from build123d import *

# Parameters (mm, degrees)
BOSS_EXTRUDE1_DEPTH = 101.6
CUT_EXTRUDE1_START  = -25.4
SKETCH3_W           = 165.1
SKETCH3_H           = 76.2
CUT_EXTRUDE1_DEPTH  = 50.8
BOSS_EXTRUDE2_REACH = 306.27
SKETCH6_R           = 6.35


with BuildPart() as part:
    # Sketch1 → Boss-Extrude1 (new body)
    with BuildSketch(Plane.XY):
        with BuildLine():
            Line((0, 38.1), (254, 38.1))
            ThreePointArc((254, 38.1), (292.1, 0), (254, -38.1))
            Line((254, -38.1), (0, -38.1))
            ThreePointArc((0, -38.1), (-38.1, 0), (0, 38.1))
        make_face()
    extrude(amount=BOSS_EXTRUDE1_DEPTH)

    # Sketch3 → Cut-Extrude1 (cut)
    with BuildSketch(Plane.XY.offset(101.6).offset(CUT_EXTRUDE1_START)):
        Rectangle(SKETCH3_W, SKETCH3_H)
    cut_extrude1 = extrude(amount=-CUT_EXTRUDE1_DEPTH, mode=Mode.SUBTRACT)

    # Mirror1: Cut-Extrude1 across plane
    add(cut_extrude1.mirror(Plane(origin=(127, 0, 0), x_dir=(0, 0, 1), z_dir=(1, 0, 0))), mode=Mode.SUBTRACT)

    # Sketch6 → Boss-Extrude2 (add, up to next)
    with BuildSketch(Plane.XY.offset(25.4), mode=Mode.PRIVATE) as boss_extrude2_sk1:
        with Locations(Location((0, 0, 0), (0, 0, 180))):
            Circle(SKETCH6_R)
    boss_extrude2_tool1 = extrude(boss_extrude2_sk1.sketch, amount=BOSS_EXTRUDE2_REACH, mode=Mode.PRIVATE) - part.part
    boss_extrude2 = boss_extrude2_tool1.solids().sort_by_distance((0, 0, 25.4))[0]
    add(boss_extrude2)

    # Mirror2: Boss-Extrude2 across plane
    add(boss_extrude2.mirror(Plane(origin=(127, 0, 0), x_dir=(0, 0, 1), z_dir=(1, 0, 0))))


solid = part.part
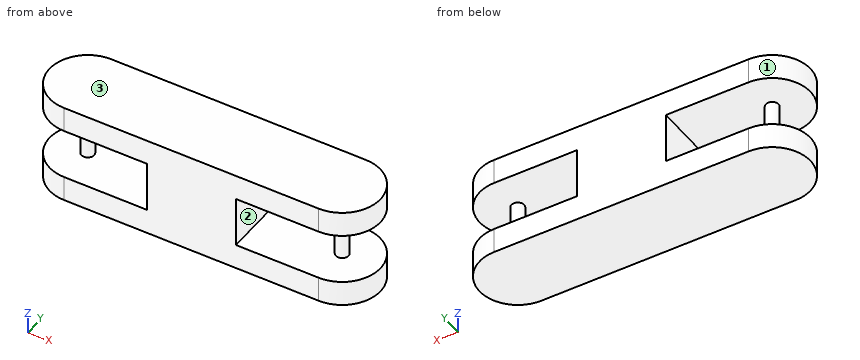
Geometry check sheet. Reference: the model listing, model coordinates, mm. Face numbers are marked on the shaded views. Round coordinates to 2 decimals unless told otherwise and drop trailing zeros. Order: outer loops, then holes, each group sorted by start corner. A loop starts at its lowest first (then second) coordinate and runs counter-clockwise, first axis right, second up. Notation, with made-up numbers: M -14,29 L 45,29 A12 cw 45,48 Z; hole C 73.25,33.25 d3. An arc over 180 degrees is marked long. Write each question's results on one line, items separated by ' | '. Start each with the question number.
1. Cross-section at C-C on z = 29. Record the boundary of the cut face in (x, y), plus the area to 3 significant figures.
2. Cross-section at B-B on y = 0. Record the boundary of the cut face in (x, z), plus the area to 3 significant figures.
3. Material ranges on L1, parallel to Z at x = 50, y = -4; L2, parallel to X at y = 4, z = 72; L3, parallel to X at y = -14, z = 44, recorded low to high. Write a range as from..to.
4. Cross-section at A-A on x = 183. Record the boundary of the cut face in (y, z), plus the area to 3 significant figures.
5. Draft check along Z on the marked faces 1, 2 and 3. Enter one of: pulls with the +Z half, pulls with the -Z half, needs draft (parallel to the pull), parting line crosses it, or undercut.
6. Cross-section at D-D on y = 13. Record the boundary of the cut face in (x, z), plus the area to 3 significant figures.
7. Go/stop test with flat-tipped pins: P1, Ø1.5, axis at y = 0, z = 70, coming from the -X side; P2, Ø5, axis at y = 23, z = 31, coming from the +X side; P3, Ø10, axis at y = 6.5, z = 81.5, coming from the -X side. Record where each tip stops, or that it passes through.
Resolved:
1) outline: C 0,0 d12.7; M 82.55,-38.1 L 171.45,-38.1 L 171.45,38.1 L 82.55,38.1 Z; C 254,0 d12.7 | area: 7,030 mm2
2) outline: M -38.1,0 L 292.1,0 L 292.1,25.4 L 260.35,25.4 L 260.35,76.2 L 292.1,76.2 L 292.1,101.6 L -38.1,101.6 L -38.1,76.2 L -6.35,76.2 L -6.35,25.4 L -38.1,25.4 Z; hole M 6.35,25.4 L 82.55,25.4 L 82.55,76.2 L 6.35,76.2 Z; hole M 171.45,25.4 L 247.65,25.4 L 247.65,76.2 L 171.45,76.2 Z | area: 22,600 mm2
3) L1: 0..25.4, 76.2..101.6 | L2: -4.93..4.93, 82.55..171.45, 249.07..258.93 | L3: 82.55..171.45
4) outline: M -38.1,0 L 38.1,0 L 38.1,25.4 L -38.1,25.4 Z; M -38.1,76.2 L 38.1,76.2 L 38.1,101.6 L -38.1,101.6 Z | area: 3,870 mm2
5) face 1: needs draft | face 2: undercut | face 3: pulls with the +Z half
6) outline: M -35.81,0 L 289.81,0 L 289.81,25.4 L 171.45,25.4 L 171.45,76.2 L 289.81,76.2 L 289.81,101.6 L -35.81,101.6 L -35.81,76.2 L 82.55,76.2 L 82.55,25.4 L -35.81,25.4 Z | area: 21,100 mm2
7) P1: x = -6.35 | P2: x = 171.45 | P3: x = -38.07
